The listing builds one solid part. Answer for the finished solid, in the listing's coordinates (mm). A direction names the side the tool comes from. Round coordinates to 2 decimals unless told otherwise and drop trailing zeros. Order: outer loops, then holes, each group sorted by start corner. A loop starts at its lowest first (then second) coordinate and runs counter-clockwise, first axis right, second up. Notation, with made-up numbers: (70, 53) - (122, 53) arc R13 cw to (122, 60) - close; hole circle Ø6 at (-24, -28). An arc over 180 degrees is marked (long way). One line per item, written item: value. Start each with the question number.
1. Section C-C, the plane z = 14.75 is taken. Give the vertices of the cut face in (x, y).
2. Flat-ended cylindrical pins translate along their axes: P1, Ø1, axis at y = -0.5, z = 9, coming from the +X side (3 decimals); P2, Ø10, axis at y = 3, z = 3, coming from the -X side (3 decimals). Find the tip coordinate at first contact, or state that the pin passes through.
3. For a pull along Y with two mould halves and no side action, classify faces 3 (the cylindrical face through (-0.13, 0.45, 17.31)), 4 (the flat face through (-4, 6, 12.52)), 5 (the flat face through (0, -9.5, 19)) as released by +Y, released by -Y, zero draft, split by the parting line, or undercut.
4. Section B-B, the plane x = 0 is taken. Give the vertices of the cut face in (y, z) (3 decimals), then the cut area to 3 significant figures.
5. Section D-D, the plane y = -2.75 is taken. Give the vertices of the cut face in (x, z), then the cut area to 3 significant figures.
6. Section A-A, the plane y = 0 is taken. Give the vertices of the cut face in (x, z) (3 decimals), then the cut area to 3 significant figures.
7. A tool of negligible diameter and unlimited length cuts with its end or side. For faces 1 (the flat face through (0, 0, 0)), 2 (the cylindrical face through (-1.52, -6.86, 6.17)), from which of +Z, -Z, +X, -X, +Y, -Y can it reach the whole face along a straight path? Write none if from no direction.
8. Straight lines are drawn through the part: line 1 (Y direction, x = -5.5, z = 15.88); line 2 (Y direction, x = 1.5, z = 16.75); line 3 (Z direction, x = 8.75, y = 1.75). For each, find the intervals that lie inside material, in ascending order.
from build123d import *

# Parameters (mm, degrees)
SKETCH_1_R          = 7.025
EXTRUDE_1_DEPTH     = 12.52
SKETCH_2_W          = 19
SKETCH_2_H          = 19
EXTRUDE_2_DEPTH     = 14
SKETCH_3_R          = 1.5
CUT_EXTRUDE_1_DEPTH = 34.978822817


with BuildPart() as part:
    # 草图1 → 凸台-拉伸1 (new body)
    with BuildSketch(Plane.XY):
        Circle(SKETCH_1_R)
    extrude(amount=EXTRUDE_1_DEPTH)

    # 草图2 → 凸台-拉伸2 (add)
    with BuildSketch(Plane.XY.offset(12.52)):
        Rectangle(SKETCH_2_W, SKETCH_2_H)
    extrude(amount=EXTRUDE_2_DEPTH)

    # 草图3 → 切除-拉伸1 (cut, through all)
    with BuildSketch(Plane.ZY.offset(9.5)):
        with Locations((15.88, 0)):
            Circle(SKETCH_3_R)
    extrude(amount=-CUT_EXTRUDE_1_DEPTH, mode=Mode.SUBTRACT)


solid = part.part
Answer list:
1. outline: (-9.5, -9.5) - (9.5, -9.5) - (9.5, -0.99) - (-9.5, -0.99) - close; (-9.5, 0.99) - (9.5, 0.99) - (9.5, 9.5) - (-9.5, 9.5) - close
2. P1: stops at x = 7.025
2. P2: stops at x = -7.025
3. face 3: undercut
3. face 4: zero draft
3. face 5: released by -Y
4. outline: (-9.5, 12.52) - (-7.025, 12.52) - (-7.025, 0) - (7.025, 0) - (7.025, 12.52) - (9.5, 12.52) - (9.5, 26.52) - (-9.5, 26.52) - close; hole circle Ø3 at (0, 15.88)
4. area: 435 mm²
5. outline: (-9.5, 12.52) - (-6.46, 12.52) - (-6.46, 0) - (6.46, 0) - (6.46, 12.52) - (9.5, 12.52) - (9.5, 26.52) - (-9.5, 26.52) - close
5. area: 428 mm²
6. outline: (-9.5, 12.52) - (-7.025, 12.52) - (-7.025, 0) - (7.025, 0) - (7.025, 12.52) - (9.5, 12.52) - (9.5, 14.38) - (-9.5, 14.38) - close; (-9.5, 17.38) - (9.5, 17.38) - (9.5, 26.52) - (-9.5, 26.52) - close
6. area: 385 mm²
7. face 1: -Z, +X, -X, +Y, -Y
7. face 2: -Z
8. line 1: y = -9.5 to -1.5, 1.5 to 9.5
8. line 2: y = -9.5 to -1.22, 1.22 to 9.5
8. line 3: z = 12.52 to 26.52
